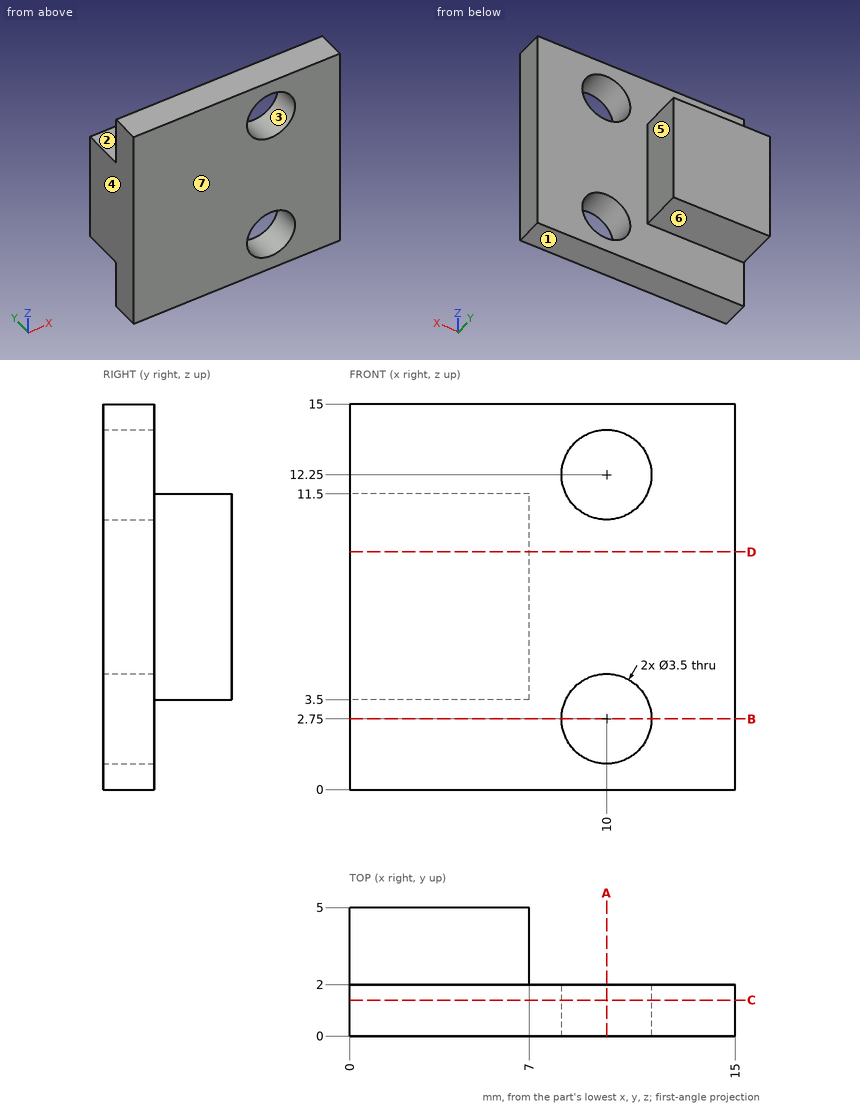
Check sheet for the drawn part. Datum: minimum x, y, z corner. Units: mm. A direction names the side the tool comes from. Round coordinates to 2 decimals unless told otherwise and drop trailing zeros. Loops run counter-clockwise (first coordinate to the right, second up) from the corner with the lowest first, then second, coordinate; pieces in that order, holes last. Notation, with made-up numbers: (0.25, 34.5) - (51.25, 34.5) arc R17 cw to (51.25, 47.5) - close; hole circle Ø8 at (10, 1). An arc over 180 degrees is marked (long way). Write each question's results on one line, items separated by ' | '. Start each with the question number.
Q1. Cross-section at B-B on z = 2.75. Enter the section's corners in (x, y).
Q2. Gauge pin test, flat ends, axial feed: P1, Ø4.5, axis at x = 10, z = 2.75, coming from the +Y side; P2, Ø1.5, axis at x = 4.5, y = 4, coming from the -Z side; P3, Ø0.9, axis at x = 3, y = 3, coming from the +Z side; P4, Ø3, axis at x = 10, z = 12.25, coming from the -Y side. Record the tip position at first contact, or that the pin passes through.
Q3. Thickness scan on line 1 (Z direction, x = 10, y = 0.95); line 2 (X direction, y = 0.8, z = 12.25); line 3 (Z direction, x = 8.75, y = 1.95). Record the ranges inside material, lowest first. Write a range as [from, to].
Q4. Cross-section at A-A on x = 10. Enter the section's corners in (y, z), and give its area (3 significant figures).
Q5. Release check for a two-part mould opening along Z. For the marked faces 1, 2, 3 and 4 record: +Z half, -Z half, draft (parallel to the pull), parting line (faces both ways), or undercut.
Q6. Cross-section at D-D on z = 9.25. Enter the section's corners in (x, y), and give its area (3 significant figures).
Q7. Access from +Z, -Z, +X, -X, +Y, -Y to the whole of each face (thin tool, end or side, straight path). Record for the marked faces 5, 6 and 7.
Q8. Cross-section at C-C on y = 1.4. Enter the section's corners in (x, z), and give its area (3 significant figures).
Answers below:
1) outline: (0, 0) - (8.25, 0) - (8.25, 2) - (0, 2) - close; (11.75, 0) - (15, 0) - (15, 2) - (11.75, 2) - close
2) P1: stops at y = 2 | P2: stops at z = 3.5 | P3: stops at z = 11.5 | P4: passes through
3) line 1: z = [0, 1], [4.5, 10.5], [14, 15] | line 2: x = [0, 8.25], [11.75, 15] | line 3: z = [0, 1.53], [3.97, 11.03], [13.47, 15]
4) outline: (0, 0) - (2, 0) - (2, 1) - (0, 1) - close; (0, 4.5) - (2, 4.5) - (2, 10.5) - (0, 10.5) - close; (0, 14) - (2, 14) - (2, 15) - (0, 15) - close | area: 16.0 mm²
5) face 1: -Z half | face 2: +Z half | face 3: undercut | face 4: draft
6) outline: (0, 0) - (15, 0) - (15, 2) - (7, 2) - (7, 5) - (0, 5) - close | area: 51.0 mm²
7) face 5: +Z, -Z, +X, +Y | face 6: -Z, +X, -X, +Y | face 7: +Z, -Z, +X, -X, -Y
8) outline: (0, 0) - (15, 0) - (15, 15) - (0, 15) - close; hole circle Ø3.5 at (10, 2.75); hole circle Ø3.5 at (10, 12.25) | area: 206 mm²
